Read the model definition and answer for the solid it produces. Units are mm, in the model's axes. Face numbers are marked on the shaded views. A direction names the side the tool comes from. Give positions to 0.01 mm unless a question says otherwise; leave off trailing zeros. Order: outer loops, then holes, each group sorted by start corner. A loop starts at its lowest first (then second) coordinate and runs counter-clockwise, first axis right, second up. Notation, with made-up numbers: (-26, 1) - (26, 1) arc R13 ccw to (26, 23) - close; hole circle Ø7 at (6, 22). An arc over 180 degrees is marked (long way). One line per item, written item: value. Start each with the question number.
```python
from build123d import *

# Parameters (mm, degrees)
BOSS_EXTRUDE1_DEPTH = 2.4
BOSS_EXTRUDE2_DEPTH = 9
SKETCH2_R           = 2.150011747
BOSS_EXTRUDE3_DEPTH = 9
CUT_EXTRUDE1_DEPTH  = 10


with BuildPart() as part:
    # Sketch1 → Boss-Extrude1 (new body)
    with BuildSketch(Plane(origin=(0, 0, 0), x_dir=(1, 0, 0), z_dir=(0, 1, 0))):
        with BuildLine():
            Line((-39.556221528, -6.891215643), (-5.823918226, -16.078704856))
            ThreePointArc((-5.823918226, -16.078704856), (21.515277807, 0.00207027), (-5.827536633, 16.076692097))
            Line((-5.827536633, 16.076692097), (-39.556221528, 6.891215643))
            Line((-39.556221528, 6.891215643), (-48.371159118, 10.670216357))
            ThreePointArc((-48.371159118, 10.670216357), (-67.382417284, 0), (-48.371159118, -10.670216357))
            Line((-48.371159118, -10.670216357), (-39.556221528, -6.891215643))
        make_face()
        with BuildLine():
            Line((-8.122758878, -10.441521159), (-8.105229312, -11.643301988))
            Line((-8.105229312, -11.643301988), (-28.234913418, -6.160686291))
            Line((-28.234913418, -6.160686291), (-28.234913418, -3.434881235))
            Line((-28.234913418, -3.434881235), (-26.602273601, -3.879554715))
            Line((-26.602273601, -3.879554715), (-10.183921919, -8.35133441))
            ThreePointArc((-10.183921919, -8.35133441), (-9.210480376, -9.452774334), (-8.122758878, -10.441521159))
        make_face(mode=Mode.SUBTRACT)
        with BuildLine():
            Line((-28.234913418, 6.161641155), (-8.104625251, 11.643808294))
            Line((-8.104625251, 11.643808294), (-8.119473087, 10.444385808))
            ThreePointArc((-8.119473087, 10.444385808), (-9.209489158, 9.453970662), (-10.184798219, 8.350417567))
            Line((-10.184798219, 8.350417567), (-26.60206646, 3.879432964))
            Line((-26.60206646, 3.879432964), (-28.234913418, 3.434752795))
            Line((-28.234913418, 3.434752795), (-28.234913418, 6.161641155))
        make_face(mode=Mode.SUBTRACT)
        with BuildLine():
            Line((-4.336944207, -12.669649891), (-6.180251244, -12.167598093))
            Line((-6.180251244, -12.167598093), (-6.180251244, -11.758725803))
            ThreePointArc((-6.180251244, -11.758725803), (13.838310708, -0.01960386), (-6.145811005, 11.778052091))
            Line((-6.145811005, 11.778052091), (-6.145811005, 12.177260522))
            Line((-6.145811005, 12.177260522), (-4.336225757, 12.670072583))
            ThreePointArc((-4.336225757, 12.670072583), (17.81758271, -0.000416785), (-4.336944207, -12.669649891))
        make_face(mode=Mode.SUBTRACT)
    extrude(amount=BOSS_EXTRUDE1_DEPTH)



with BuildPart() as body_2:
    # Sketch1<4> → Boss-Extrude2 (new body)
    with BuildSketch(Plane(origin=(0, 0, 0), x_dir=(1, 0, 0), z_dir=(0, 1, 0))):
        with BuildLine():
            ThreePointArc((-57.032417284, 0), (-54.882417284, -2.15), (-52.732417284, 0))
            Line((-52.732417284, 0), (-57.032417284, 0))
        make_face()
        with BuildLine():
            Line((-57.032417284, 0), (-52.732417284, 0))
            ThreePointArc((-52.732417284, 0), (-54.882417284, 2.15), (-57.032417284, 0))
        make_face()
    extrude(amount=-BOSS_EXTRUDE2_DEPTH)


with BuildPart() as part_1:
    add(part.part)

    add(body_2.part)  # Boss-Extrude3 merges body 2
    # Sketch2 → Boss-Extrude3 (add)
    with BuildSketch(Plane(origin=(0, 2.4, 0), x_dir=(1, 0, 0), z_dir=(0, 1, 0))):
        with Locations((-54.882419847, 1.1464e-05)):
            Circle(SKETCH2_R)
    extrude(amount=-BOSS_EXTRUDE3_DEPTH)

    # Sketch3 → Cut-Extrude1 (cut)
    with BuildSketch(Plane(origin=(0, 2.4, 0), x_dir=(1, 0, 0), z_dir=(0, 1, 0))):
        with BuildLine():
            ThreePointArc((-48.415945495, 6.259771763), (-54.736258294, 8.998813115), (-61.142189047, 6.466471789))
            Line((-61.142189047, 6.466471789), (-59.751128654, 5.029478057))
            ThreePointArc((-59.751128654, 5.029478057), (-54.768738069, 6.999076866), (-49.852939226, 4.86871137))
            Line((-49.852939226, 4.86871137), (-48.415945495, 6.259771763))
        make_face()
        with BuildLine():
            Line((-59.911895341, -4.86871137), (-61.348889073, -6.259771763))
            ThreePointArc((-61.348889073, -6.259771763), (-55.028576274, -8.998813115), (-48.622645521, -6.466471789))
            Line((-48.622645521, -6.466471789), (-50.013705914, -5.029478057))
            ThreePointArc((-50.013705914, -5.029478057), (-54.996096499, -6.999076866), (-59.911895341, -4.86871137))
        make_face()
    extrude(amount=-CUT_EXTRUDE1_DEPTH, mode=Mode.SUBTRACT)


solid = part_1.part
```
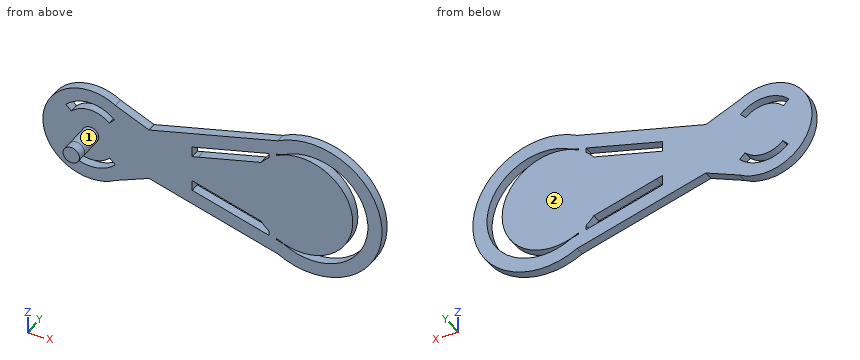
1) Section A-A on x = -17 is taken. Write down the section's boundary in (y, z).
2) Each of these flat-tipped pins is pushed along its axis until it touches: pin 1 (6 mm diameter, centred on y = -1.5, z = -14.5, fed in from +X); pin 2 (2.5 mm diameter, centred on y = 0.5, z = -5, fed in from +X); pin 3 (5 mm diameter, centred on x = -21, z = 5, fed in from -Y). Where does it stop, or does it pass through?
3) Section B-B on x = -1 is taken. Write down the section's boundary in (y, z), plus the area to 3 significant figures.
4) Find the intervals of material crossed by probe 1 along Y at (x, z) = (-27, 10); probe 2 along X at (y, z) = (0.25, 2.5); probe 3 along X at (y, z) = (0.5, -17), in increasing order. Write a range as from..to.
5) Section C-C on y = -4.75 is taken. Write down the section's boundary in (x, z), plus the area to 3 significant figures.
6) For the marked faces 1 and 2, determine the directions among +Z, -Z, +X, -X, +Y, -Y from which every point of the face is accessible in a straight line to the end or side of a thin tool.
Solved:
1. outline: (0, -13.03) - (2.4, -13.03) - (2.4, -9.22) - (0, -9.22) - close; (0, -6.49) - (2.4, -6.49) - (2.4, 6.49) - (0, 6.49) - close; (0, 9.22) - (2.4, 9.22) - (2.4, 13.03) - (0, 13.03) - close
2. pin 1: stops at x = 17.15
2. pin 2: stops at x = 21.13
2. pin 3: stops at y = 0
3. outline: (0, -17.93) - (2.4, -17.93) - (2.4, -14.11) - (0, -14.11) - close; (0, -13.39) - (2.4, -13.39) - (2.4, 13.39) - (0, 13.39) - close; (0, 14.11) - (2.4, 14.11) - (2.4, 17.93) - (0, 17.93) - close
3. area: 82.6 mm2
4. probe 1: y = 0..2.4
4. probe 2: x = -67.13..13.6, 17.6..21.34
4. probe 3: x = -3.92..10.15
5. outline: circle Ø4.3 at (-54.88, 0)
5. area: 14.5 mm2
6. face 1: -Y
6. face 2: +Z, -Z, +X, -X, +Y
